For this review, take the finished solid that the model builds, in its own axes (mm). Face numbers are marked on the shaded views. A direction names the side the tool comes from. Round coordinates to 2 decimals unless told otherwise and drop trailing zeros. Loops run counter-clockwise (first coordinate to the right, second up) from the corner with the lowest first, then second, coordinate; pieces in that order, holes last.
1. Draft analysis for pull direction X (two halves, no side actions). For the marked faces 1, 2, 3 and 4, state which applies: released by +X, released by -X, zero draft, split by the parting line, or undercut.
2. Consider section A-A on y = 50. State the section outline as (x, z) points.
3. Consider section C-C on z = 33.5. State the section outline as (x, y) points.
4. To check wall thickness, follow line 1 along Y through (x, z) = (50, 138.5); line 2 along Y through (x, z) = (50, 153.5); line 3 along X through (y, z) = (-75, 186). State the ranges of each line that lie inside material, in increasing order.
5. Consider section D-D on z = 143. State the section outline as (x, y) points.
6. Consider section B-B on x = -50. State the section outline as (y, z) points, then the cut area to 3 significant figures.
7. Tool access review of the marked faces 5 and 6: name each direction out of +Z, -Z, +X, -X, +Y, -Y from which nothing blocks a thin tool from reaching the whole face with its end or side.
from build123d import *

# Parameters (mm, degrees)
SKETCH_W     = 200
SKETCH_H     = 200
SKETCH_R     = 30
PAD_DEPTH    = 200
SKETCH001_R  = 30
POCKET_DEPTH = 100
SKETCH002_R  = 30
SKETCH003_R  = 10
SKETCH004_R  = 30
SKETCH005_R  = 10


with BuildPart() as part:
    # Sketch → Pad (new body)
    with BuildSketch(Plane.XY):
        Rectangle(SKETCH_W, SKETCH_H)
        with Locations((50, 50)):
            Circle(SKETCH_R, mode=Mode.SUBTRACT)
    extrude(amount=PAD_DEPTH)

    # Sketch001 (on Face7 of Pad) → Pocket (cut)
    with BuildSketch(Plane.XY.offset(200)):
        with Locations((-50, 50)):
            Circle(SKETCH001_R)
    extrude(amount=-POCKET_DEPTH, mode=Mode.SUBTRACT)

    # Sketch002 (on Face5 of Pocket) → SubtractiveLoft section 0
    with BuildSketch(Plane.XY.offset(200)):
        with Locations((-50, -50)):
            Circle(SKETCH002_R)
    # Sketch003 (on Face4 of Pocket) → SubtractiveLoft section 1
    with BuildSketch(Plane(origin=(0, 0, 0), x_dir=(1, 0, 0), z_dir=(0, 0, -1))):
        with Locations((-50, 50)):
            Circle(SKETCH003_R)
    loft(mode=Mode.SUBTRACT)

    # Sketch004 (on Face5 of SubtractiveLoft) → SubtractiveLoft001 section 0
    with BuildSketch(Plane.XY.offset(200)):
        with Locations((50, -50)):
            Circle(SKETCH004_R)
    # Sketch005 (on Face4 of SubtractiveLoft) → SubtractiveLoft001 section 1
    with BuildSketch(Plane(origin=(0, 0, 50), x_dir=(1, 0, 0), z_dir=(0, 0, -1))):
        with Locations((50, 50)):
            Circle(SKETCH005_R)
    loft(mode=Mode.SUBTRACT)


solid = part.part
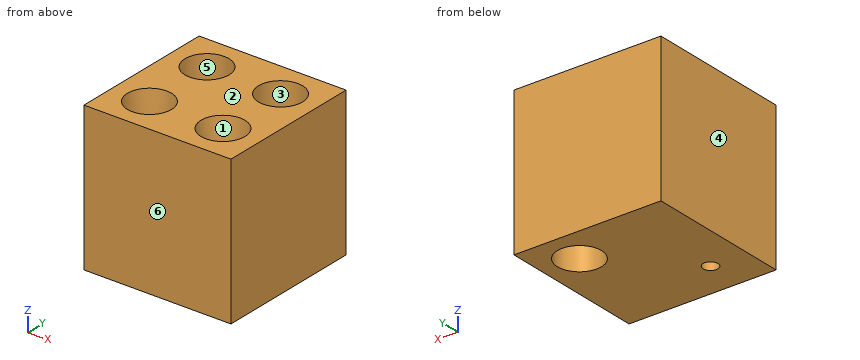
Resolved:
1. face 1: undercut
1. face 2: zero draft
1. face 3: undercut
1. face 4: released by -X
2. outline: (-100, 0) - (20, 0) - (20, 200) - (-20, 200) - (-20, 100) - (-80, 100) - (-80, 200) - (-100, 200) - close; (80, 0) - (100, 0) - (100, 200) - (80, 200) - close
3. outline: (-100, -100) - (100, -100) - (100, 100) - (-100, 100) - close; hole circle Ø26.7 at (-50, -50); hole circle Ø60 at (50, 50)
4. line 1: y = -100 to -71.8, -28.2 to 20, 80 to 100
4. line 2: y = -100 to -73.8, -26.2 to 20, 80 to 100
4. line 3: x = -100 to -63.89, -36.11 to 37.1, 62.9 to 100
5. outline: (-100, -100) - (100, -100) - (100, 100) - (-100, 100) - close; hole circle Ø60 at (-50, 50); hole circle Ø48.6 at (-50, -50); hole circle Ø60 at (50, 50); hole circle Ø44.8 at (50, -50)
6. outline: (-100, 0) - (-60, 0) - (-80, 200) - (-100, 200) - close; (-40, 0) - (100, 0) - (100, 200) - (80, 200) - (80, 100) - (20, 100) - (20, 200) - (-20, 200) - close
6. area: 26,000 mm2
7. face 5: +Z
7. face 6: +Z, -Z, +X, -X, -Y
